Solid Edge part; units mm, degrees
sketch "Sketch1" plane through (0, 0, 0) normal (0, 0, 1) x (1, 0, 0)
  line L0 (-69.2032, 20.9413) -> (-19.2032, 20.9413)
  line L1 (-19.2032, 20.9413) -> (-19.2032, 70.9413)
  line L2 (-19.2032, 70.9413) -> (-69.2032, 70.9413)
  line L3 (-69.2032, 70.9413) -> (-69.2032, 20.9413)
extrude "Protrusion1" add sketch "Sketch1" along normal blind 70
sketch "Sketch2" plane through (-19.2032, 45.9413, 5) normal (1, 0, 0) x (0, 1, 0)
  line L0 (-25, 65) -> (25, 65)
  line L1 (25, 65) -> (25, 85)
  line L2 (25, 85) -> (-25, 85)
  line L3 (-25, 85) -> (-25, 65)
  dimension "D1" = 25
  dimension "D2" = 25
extrude "ExtrudedProtrusion_2" add sketch "Sketch2" against normal blind 5
sketch "Sketch3" plane through (-44.2032, 20.9413, 30) normal (0, -1, 0) x (1, 0, 0)
  line L0 (17.1738, 55) -> (25.8341, 60)
  line L1 (25.8341, 60) -> (20.8341, 68.6602)
  line L2 (20.8341, 68.6602) -> (12.1738, 63.6602)
  line L3 (12.1738, 63.6602) -> (17.1738, 55)
  dimension "D1" = 20.8341
  dimension "D2" = 12.1738
extrude "Cutout1" cut sketch "Sketch3" against normal through all
mirror "Mirror1" about plane through (-44.2032, 45.9413, 30) normal (1, 0, 0) of "ExtrudedProtrusion_2", "Cutout1"
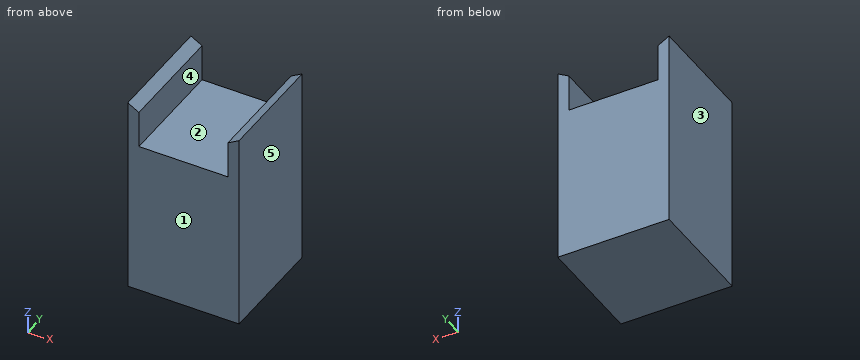
The model under review builds one solid part; all positions refer to its coordinate system, in mm. Face numbers are marked on the shaded views. A direction names the side the tool comes from. Give positions to 0.01 mm unless a question says otherwise; leave off trailing zeros. Write each loop counter-clockwise with the first axis right and the second up, starting at its lowest first coordinate (ties: lowest second). Pieces come first, ordered by that corner, then holes.
1. Add section A-A, the plane z = 82.5. Write out the cut boundary in (x, y), plus the area to 3 significant figures.
2. For P1, Ø3, axis at x = -24.5, y = 51, coming from the +Z side; P2, Ø4, axis at x = -26.5, y = 45, coming from the +Z side; P3, Ø3, axis at x = -52, y = 60, coming from the -Z side, all flat-tipped, find the tip position at first contact; note any pin that passes through.
3. Tool access review of the marked faces 1 and 2: name each direction out of +Z, -Z, +X, -X, +Y, -Y from which nothing blocks a thin tool from reaching the whole face with its end or side.
4. Draft analysis for pull direction X (two halves, no side actions). For the marked faces 3, 4 and 5, state which applies: +X half, -X half, draft (parallel to the pull), parting line (faces both ways), or undercut.
5. Add section B-B, the plane y = 57. Write out the cut boundary in (x, z).
6. Add section C-C, the plane x = -35.5. Write out the cut boundary in (y, z).
7. Wall thickness on L1, parallel to X at y = 54, z = 79.5; L2, parallel to Z at x = -48.5, y = 57; L3, parallel to Z at x = -66, y = 65: over which ranges is each line inside the solid? List them lowest first.
Worked answers:
1. outline: (-69.2, 20.94) - (-64.2, 20.94) - (-64.2, 70.94) - (-69.2, 70.94) - close; (-24.2, 20.94) - (-19.2, 20.94) - (-19.2, 70.94) - (-24.2, 70.94) - close
1. area: 500 mm2
2. P1: stops at z = 87.33
2. P2: stops at z = 70
2. P3: stops at z = 0
3. face 1: +Z, -Z, +X, -X, -Y
3. face 2: +Z, +Y, -Y
4. face 3: -X half
4. face 4: undercut
4. face 5: +X half
5. outline: (-69.2, 0) - (-19.2, 0) - (-19.2, 89.52) - (-24.2, 86.63) - (-24.2, 70) - (-64.2, 70) - (-64.2, 86.63) - (-69.2, 89.52) - close
6. outline: (20.94, 0) - (70.94, 0) - (70.94, 70) - (20.94, 70) - close
7. L1: x = -69.2 to -64.2, -24.2 to -19.2
7. L2: z = 0 to 70
7. L3: z = 0 to 87.67
